Could you check a few things on this model? Use its own coordinates, in mm. Face numbers are marked on the shaded views. Give positions to 0.01 mm unless a question says otherwise; leave off trailing zeros. Order: outer loops, then holes, each group sorted by start corner. A loop starts at its lowest first (then second) coordinate and runs counter-clockwise, first axis right, second up. Notation, with made-up numbers: (-15.5, 11) -> (7.5, 11) arc R28 ccw to (7.5, 34) -> close; hole circle Ø4 at (65, 71). An arc over 180 degrees is marked (long way). Answer as CSV lines item,"result". Start each with the question number.
(1) I want a section at D-D (x = 3.25). Please give me the cut outline in (y, z), plus the area to 3 significant figures.
(2) I want a section at C-C (z = 21). Please give me the cut outline in (x, y), plus the area to 3 significant figures.
(3) I want a section at B-B (y = 0). Please give me the cut outline in (x, z), plus the area to 3 significant figures.
(4) I want a section at A-A (x = 0). Please give me the cut outline in (y, z), plus the area to 3 significant figures.
(5) Will these pins go through, and if not, where does the flat tip stop? pin 1 Ø2 at (x, z) = (0, 38) entering from +Y; pin 2 Ø1 at (x, z) = (1.5, 10) entering from +Y; pin 3 Ø1.7 at (y, z) = (5, 36) entering from +X.
(6) I need wall thicknesses on L1, parallel to X at y = -0.25, z = 30; L2, parallel to X at y = -2.25, z = 26; L3, parallel to Y at x = 2, z = 43.5. Which ranges of each line are inside material? Lowest first, please.
(7) We'd pull the mould along X, two halves only. Please class the marked faces 1 and 2: released by +X, released by -X, zero draft, split by the parting line, or undercut.
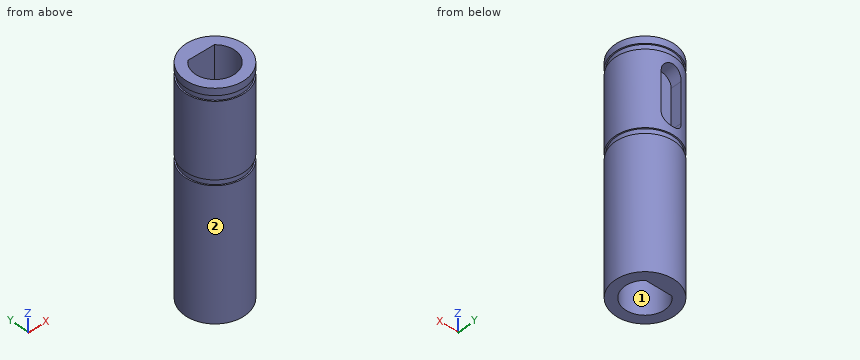
```python
from build123d import *

# Parameters (mm, degrees)
ESBO_O1_R                = 6
RESSALTO_EXTRUS_O1_DEPTH = 45
CORTE_EXTRUS_O1_DEPTH    = 2.5
ESBO_O3_W                = 1.1
ESBO_O3_H                = 0.25


with BuildPart() as part:
    # Esboço1 → Ressalto-extrusão1 (new body)
    with BuildSketch(Plane.XY):
        with Locations(Location((0, 0, 0), (0, 0, 180))):
            Circle(ESBO_O1_R)
        with BuildLine():
            Line((-2.645751311, 3), (2.645751311, 3))
            ThreePointArc((2.645751311, 3), (0, -4), (-2.645751311, 3))
        make_face(mode=Mode.SUBTRACT)
    extrude(amount=RESSALTO_EXTRUS_O1_DEPTH)

    # Esboço2 → Corte-extrusão1 (cut)
    with BuildSketch(Plane(origin=(0, 6, 0), x_dir=(1, 0, 0), z_dir=(0, 1, 0))):
        with BuildLine():
            Line((-2, -39), (-2, -31))
            ThreePointArc((-2, -31), (0, -29), (2, -31))
            Line((2, -31), (2, -39))
            ThreePointArc((2, -39), (0, -41), (-2, -39))
        make_face()
    extrude(amount=-CORTE_EXTRUS_O1_DEPTH, mode=Mode.SUBTRACT)

    # Esboço3 → Corte-Revolução1 (revolve, cut)
    with BuildSketch(Plane(origin=(0, 0, 0), x_dir=(0, 0, -1), z_dir=(1, 0, 0)), mode=Mode.PRIVATE) as corte_revolu_o1_sk:
        with Locations((-26.95, 5.875)):
            Rectangle(ESBO_O3_W, ESBO_O3_H)
        with Locations((-43.05, 5.875)):
            Rectangle(ESBO_O3_W, ESBO_O3_H)
    revolve(corte_revolu_o1_sk.sketch.rotate(Axis((0, 0, 0), (0, 0, 1)), 90), axis=Axis((0, 0, 0), (0, 0, 1)), mode=Mode.SUBTRACT)


solid = part.part
```
Final values:
1,outline,"(-5.04, 0) -> (-2.33, 0) -> (-2.33, 45) -> (-5.04, 45) -> (-5.04, 43.6) -> (-4.74, 43.6) -> (-4.74, 42.5) -> (-5.04, 42.5) -> (-5.04, 27.5) -> (-4.74, 27.5) -> (-4.74, 26.4) -> (-5.04, 26.4) -> close; (2.33, 0) -> (5.04, 0) -> (5.04, 26.4) -> (4.74, 26.4) -> (4.74, 27.5) -> (5.04, 27.5) -> (5.04, 42.5) -> (4.74, 42.5) -> (4.74, 43.6) -> (5.04, 43.6) -> (5.04, 45) -> (2.33, 45) -> close"
1,area,"243 mm²"
2,outline,"circle Ø12 at (0, 0); hole (-2.65, 3) arc R4 ccw (long way) to (2.65, 3) -> close"
2,area,"66.5 mm²"
3,outline,"(-6, 0) -> (-4, 0) -> (-4, 45) -> (-6, 45) -> (-6, 43.6) -> (-5.75, 43.6) -> (-5.75, 42.5) -> (-6, 42.5) -> (-6, 27.5) -> (-5.75, 27.5) -> (-5.75, 26.4) -> (-6, 26.4) -> close; (4, 0) -> (6, 0) -> (6, 26.4) -> (5.75, 26.4) -> (5.75, 27.5) -> (6, 27.5) -> (6, 42.5) -> (5.75, 42.5) -> (5.75, 43.6) -> (6, 43.6) -> (6, 45) -> (4, 45) -> close"
3,area,"179 mm²"
4,outline,"(-6, 0) -> (-4, 0) -> (-4, 45) -> (-6, 45) -> (-6, 43.6) -> (-5.75, 43.6) -> (-5.75, 42.5) -> (-6, 42.5) -> (-6, 27.5) -> (-5.75, 27.5) -> (-5.75, 26.4) -> (-6, 26.4) -> close; (3, 0) -> (6, 0) -> (6, 26.4) -> (5.75, 26.4) -> (5.75, 27.5) -> (6, 27.5) -> (6, 29) -> (3.5, 29) -> (3.5, 41) -> (6, 41) -> (6, 42.5) -> (5.75, 42.5) -> (5.75, 43.6) -> (6, 43.6) -> (6, 45) -> (3, 45) -> close"
4,area,"194 mm²"
5,pin 1,"y = 3.5"
5,pin 2,"y = 5.92"
5,pin 3,"x = 4.33"
6,L1,"-5.99 to -3.99, 3.99 to 5.99"
6,L2,"-5.56 to -3.31, 3.31 to 5.56"
6,L3,"-5.39 to -3.46, 3 to 5.39"
7,face 1,"undercut"
7,face 2,"split by the parting line"
